Model file for the job. Use its own axes, mm. Face numbers are marked on the shaded views. A direction names the side the tool comes from. Give positions to 0.01 mm unless a question says otherwise; leave off trailing zeros. Order: outer loops, then holes, each group sorted by start corner. A loop starts at its lowest first (then second) coordinate and runs counter-clockwise, first axis right, second up. Notation, with made-up numbers: M 31.5,-9 L 90.5,-9 A12 cw 90.5,10 Z; hole C 68.25,48.25 d9. An arc over 180 degrees is marked long. Return JSON: item names as keys, results as strings. Group by question number.
1. Slice it at D-D on x = -26.5. List the corners of the cut face in (y, z), then the cut area to 3 significant figures.
2. Wall check: probe 1 along X at (y, z) = (-1.75, 24); probe 2 along Z at (x, y) = (-24.25, -4.5) (1 decimal); probe 3 along Z at (x, y) = (-27.5, -4.75). Give the ranges that are in metal, low to high. Write a range as [from, to].
3. Slice it at B-B on z = 21. List the corners of the cut face in (x, y).
4. 3-axis set-ups, long thin cutter, end or side, ignore diameter. For the marked faces 4, 5 and 6: which of +Z, -Z, +X, -X, +Y, -Y reach the whole face in a straight line?
5. Two-plate mould, pull along Z, no slides. Class the marked faces 1, 2 and 3: released by +Z, released by -Z, zero draft, split by the parting line, or undercut.
6. Pin check, flat tips, straight feed: pin 1 (3 mm diameter, centred on x = -27.5, z = 13.5, fed in from +Y); pin 2 (1 mm diameter, centred on x = -29, y = -2, fed in from +Z); pin 3 (1.5 mm diameter, centred on x = -26.5, y = -3, fed in from +Z). Stop position of each tip, or through.
7. Slice it at C-C on x = -23. List the corners of the cut face in (y, z).
8. Slice it at A-A on y = -4.5. List the corners of the cut face in (x, z).
from build123d import *

# Parameters (mm, degrees)
F0_W     = 10
F0_H     = 50
F1_DEPTH = 7
F2_W     = 7
F2_H     = 20
F3_DEPTH = 5
F4_R     = 1.25
F5_DEPTH = 2.001
F7_DEPTH = 7.001


with BuildPart() as f1:
    # F0 (on Front) → F1 (new body)
    with BuildSketch(Plane.XZ):
        with Locations((-27.172005, 27.438496)):
            Rectangle(F0_W, F0_H)
    extrude(amount=F1_DEPTH)

    # F2 (on face) → F3 (cut)
    with BuildSketch(Plane(origin=(0, 0, 0), x_dir=(-1, 0, 0), z_dir=(0, 1, 0))):
        with Locations((27.172005, 14.438496)):
            Rectangle(F2_W, F2_H)
    extrude(amount=-F3_DEPTH, mode=Mode.SUBTRACT)

    # F4 (on face) → F5 (cut, through all)
    with BuildSketch(Plane(origin=(0, -5, 0), x_dir=(-1, 0, 0), z_dir=(0, 1, 0))):
        with Locations((27.172005, 8.848496)):
            Circle(F4_R)
    extrude(amount=-F5_DEPTH, mode=Mode.SUBTRACT)

    # F6 (on face) → F7 (cut, through all)
    with BuildSketch(Plane.XZ.offset(7)):
        Polygon((-32.172005, 52.438496), (-32.172005, 45.144096), (-24.652329, 52.438496), align=None)
        Polygon((-29.548446, 28.8854), (-22.172005, 25.822317), (-22.172005, 46.649169), align=None)
    extrude(amount=-F7_DEPTH, mode=Mode.SUBTRACT)


solid = f1.part
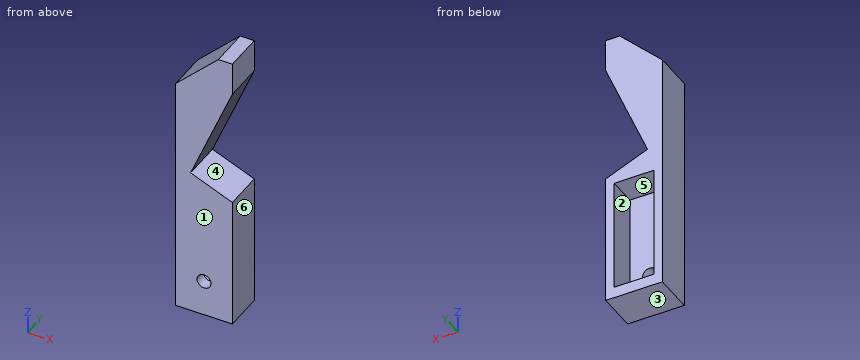
Result:
{
 "1": {"outline": "M -7,2.44 L 0,2.44 L 0,4.44 L -5,4.44 L -5,7.79 L -7,7.79 Z; M -7,9.9 L -5,9.9 L -5,24.44 L 0,24.44 L 0,27.62 L -7,27.62 Z; M -7,36.23 L 0,36.23 L 0,50.65 L -7,50.65 Z", "area": "173 mm2"},
 "2": {"probe 1": "x = [-32.17, -30.67], [-23.67, -22.17]", "probe 2": "z = [2.4, 4.4], [24.4, 26.7], [41.6, 52.4]", "probe 3": "z = [2.44, 4.44], [24.44, 28.03], [33.82, 49.68]"},
 "3": {"outline": "M -32.17,-7 L -22.17,-7 L -22.17,0 L -23.67,0 L -23.67,-5 L -30.67,-5 L -30.67,0 L -32.17,0 Z"},
 "4": {"face 4": "+X, +Y, -Y", "face 5": "+Y", "face 6": "+Z, -Z, +X, +Y, -Y"},
 "5": {"face 1": "zero draft", "face 2": "undercut", "face 3": "released by -Z"},
 "6": {"pin 1": "stops at y = -5", "pin 2": "stops at z = 48.71", "pin 3": "stops at z = 51.37"},
 "7": {"outline": "M -7,2.44 L 0,2.44 L 0,26.17 L -7,26.17 Z; M -7,44.66 L 0,44.66 L 0,52.44 L -7,52.44 Z"},
 "8": {"outline": "M -32.17,2.44 L -22.17,2.44 L -22.17,25.82 L -29.55,28.89 L -22.17,46.65 L -22.17,52.44 L -24.65,52.44 L -32.17,45.14 Z; hole M -30.67,4.44 L -23.67,4.44 L -23.67,24.44 L -30.67,24.44 Z"}
}
